Could you check a few things on this model? Use its own coordinates, in mm. A direction names the side the tool comes from. Coordinates: 2 decimals unless noted, no trailing zeros. Loops run counter-clockwise (first coordinate to the right, second up) from the corner with the lowest first, then second, coordinate; pieces in that order, holes last.
1) Imagine slicing it at C-C on z = -9.5. Please give me the cut outline in (x, y), plus the area to 3 significant figures.
2) Thinking about a two-plate mould opening in X: for faces 5 (the face through (185.502, -4.912, 1.479)), 6 (the face through (100, 38, -17)), 7 (the face through (105, 29.9, -14.4)), which applies, released by +X, released by -X, zero draft, split by the parting line, or undercut?
3) If I drill on line 1 along Y through (x, z) = (12.5, 1.3); line 2 along Z through (x, y) = (86, -4); line 3 along X through (y, z) = (22.5, -14.75), over which ranges is the centre line in solid material (lowest first)?
4) Imagine slicing it at B-B on x = 12.5. Please give me the cut outline in (y, z), plus the area to 3 significant figures.
5) For faces 1 (the face through (95, 29.9, -14.4)), 2 (the face through (10.9, -6.2, 1.5)), 3 (the face through (100, 20, -5)), 4 (the face through (100, 17, -8)), which set-ups out of +Z, -Z, +X, -X, +Y, -Y let a thin tool reach every point of the face, with its end or its side?
6) Will these pins go through, and if not, where does the flat tip stop? P1, Ø8, axis at y = 21, z = -14.5, coming from the +X side; P2, Ø10, axis at y = 15.5, z = -4.5, coming from the -X side; P3, Ø11, axis at x = 98, z = -7.5, coming from the +Y side; P4, Ø6, axis at y = 34.5, z = -8.5, coming from the +X side.
7) Imagine slicing it at A-A on y = -5. Please give me the cut outline in (x, z), plus the area to 3 significant figures.
8) Imagine slicing it at D-D on x = 97.5. Please give me the cut outline in (y, z), plus the area to 3 significant figures.
```python
from build123d import *

# Parameters (mm, degrees)
SKETCH1_W           = 200
SKETCH1_H           = 10
SKETCH1_R           = 2
BOSS_EXTRUDE1_DEPTH = 3
SKETCH2_W           = 10
SKETCH2_H           = 20
BOSS_EXTRUDE2_DEPTH = 3
SKETCH3_W           = 10
SKETCH3_H           = 3
BOSS_EXTRUDE3_DEPTH = 17
SKETCH4_W           = 10
SKETCH4_H           = 3
BOSS_EXTRUDE4_DEPTH = 40


with BuildPart() as part:
    # Sketch1 → Boss-Extrude1 (new body)
    with BuildSketch(Plane.XY):
        with Locations((100, -5)):
            Rectangle(SKETCH1_W, SKETCH1_H)
        with Locations((12.5, -5)):
            Circle(SKETCH1_R, mode=Mode.SUBTRACT)
        with Locations((187.5, -5)):
            Circle(SKETCH1_R, mode=Mode.SUBTRACT)
    extrude(amount=BOSS_EXTRUDE1_DEPTH)

    # Sketch2 → Boss-Extrude2 (add)
    with BuildSketch(Plane.XY.offset(3)):
        with Locations((100, 10)):
            Rectangle(SKETCH2_W, SKETCH2_H)
    extrude(amount=-BOSS_EXTRUDE2_DEPTH)

    # Sketch3 → Boss-Extrude3 (add)
    with BuildSketch(Plane(origin=(0, 0, 0), x_dir=(-1, 0, 0), z_dir=(0, 0, -1))):
        with Locations((-100, 18.5)):
            Rectangle(SKETCH3_W, SKETCH3_H)
    extrude(amount=BOSS_EXTRUDE3_DEPTH)

    # Sketch4 → Boss-Extrude4 (add)
    with BuildSketch(Plane(origin=(0, 20, 0), x_dir=(1, 0, 0), z_dir=(0, 1, 0))):
        with Locations((100, 15.5)):
            Rectangle(SKETCH4_W, SKETCH4_H)
    extrude(amount=BOSS_EXTRUDE4_DEPTH)


solid = part.part
```
Filled in:
1. outline: (95, 17) - (105, 17) - (105, 20) - (95, 20) - close
1. area: 30.0 mm2
2. face 5: undercut
2. face 6: zero draft
2. face 7: released by +X
3. line 1: y = -10 to -7, -3 to 0
3. line 2: z = 0 to 3
3. line 3: x = 95 to 105
4. outline: (-10, 0) - (-7, 0) - (-7, 3) - (-10, 3) - close; (-3, 0) - (0, 0) - (0, 3) - (-3, 3) - close
4. area: 18.0 mm2
5. face 1: +Z, -Z, -X, +Y
5. face 2: +Z, -Z
5. face 3: +Z, +X, -X, +Y
5. face 4: -Z, +X, -X, -Y
6. P1: stops at x = 105
6. P2: stops at x = 95
6. P3: stops at y = 20
6. P4: passes through
7. outline: (0, 0) - (10.5, 0) - (10.5, 3) - (0, 3) - close; (14.5, 0) - (185.5, 0) - (185.5, 3) - (14.5, 3) - close; (189.5, 0) - (200, 0) - (200, 3) - (189.5, 3) - close
7. area: 576 mm2
8. outline: (-10, 0) - (17, 0) - (17, -17) - (60, -17) - (60, -14) - (20, -14) - (20, 3) - (-10, 3) - close
8. area: 261 mm2
